from build123d import *

# Parameters (mm, degrees)
F0_W      = 1200
F0_H      = 400
F1_DEPTH  = 12
F2_W      = 38
F2_H      = 38
F3_DEPTH  = 128
F5_DEPTH  = 12
F7_DEPTH  = 25
F9_W      = 38
F9_H      = 38
F10_DEPTH = 120
F11_R     = 4
F12_DEPTH = 25
F13_W     = 1124
F13_H     = 324
F14_DEPTH = 25
F15_W     = 38
F15_H     = 116
F16_DEPTH = 19
F17_W     = 38
F17_H     = 116
F18_DEPTH = 19


with BuildPart() as f1:
    # F0 (on Top) → F1 (new body)
    with BuildSketch(Plane.XY):
        Rectangle(F0_W, F0_H)
    extrude(amount=F1_DEPTH)

    # F2 (on face) → F3 (join)
    with BuildSketch(Plane.XY.offset(12)):
        with Locations((-581, 181)):
            Rectangle(F2_W, F2_H)
        with Locations((581, 181)):
            Rectangle(F2_W, F2_H)
        with Locations((581, -181)):
            Rectangle(F2_W, F2_H)
        with Locations((-581, -181)):
            Rectangle(F2_W, F2_H)
    extrude(amount=F3_DEPTH)

    # F4 (on face) → F5 (join)
    with BuildSketch(Plane.XY.offset(140)):
        Polygon((600, 200), (-562, 200), (-562, 162), (-600, 162), (-600, -200), (600, -200), align=None)
    extrude(amount=-F5_DEPTH)

    # F6 (on face) → F7 (join)
    with BuildSketch(Plane.XZ.offset(200)):
        Polygon((-562, 128), (-562, 78), (-512, 128), align=None)
        Polygon((-512, 12), (-562, 62), (-562, 12), align=None)
        Polygon((562, 62), (512, 12), (562, 12), align=None)
        Polygon((562, 128), (512, 128), (562, 78), align=None)
    extrude(amount=-F7_DEPTH)

    # F8: F1 across plane


with BuildPart() as f1_1:
    add(f1.part)
    add(f1.part.mirror(Plane.XZ))

    # F9 (on face) → F10 (join)
    with BuildSketch(Plane.XY.offset(12)):
        with Locations((0, -181)):
            Rectangle(F9_W, F9_H)
        with Locations((0, 181)):
            Rectangle(F9_W, F9_H)
    extrude(amount=F10_DEPTH)

    # F11 (on face) → F12 (cut)
    with BuildSketch(Plane.XY.offset(12)):
        with Locations((-265.5, -181)):
            Circle(F11_R)
        with Locations((-581, 0)):
            Circle(F11_R)
        with Locations((-265.5, 185)):
            Circle(F11_R)
        with Locations((265.5, 181)):
            Circle(F11_R)
        with Locations((265.5, -181)):
            Circle(F11_R)
        with Locations((581, 0)):
            Circle(F11_R)
    extrude(amount=-F12_DEPTH, mode=Mode.SUBTRACT)

    # F13 (on face) → F14 (cut)
    with BuildSketch(Plane.XY.offset(140)):
        Rectangle(F13_W, F13_H)
    extrude(amount=-F14_DEPTH, mode=Mode.SUBTRACT)

    # F15 (on face) → F16 (cut)
    with BuildSketch(Plane.XZ.offset(200)):
        with Locations((0, 70)):
            Rectangle(F15_W, F15_H)
    extrude(amount=-F16_DEPTH, mode=Mode.SUBTRACT)

    # F17 (on face) → F18 (cut)
    with BuildSketch(Plane(origin=(0, 200, 0), x_dir=(-1, 0, 0), z_dir=(0, 1, 0))):
        with Locations((0, 70)):
            Rectangle(F17_W, F17_H)
    extrude(amount=-F18_DEPTH, mode=Mode.SUBTRACT)


solid = f1_1.part
Could you check a few things on this model? Use its own coordinates, in mm. A direction names the side the tool comes from. Give positions to 0.01 mm unless a question says otherwise; leave off trailing zeros. Order: outer loops, then holes, each group sorted by start corner. A loop starts at its lowest first (then second) coordinate and runs counter-clockwise, first axis right, second up. Notation, with made-up numbers: (36.25, 22.5) - (58.25, 22.5) arc R31 cw to (58.25, 47.5) - close; hole circle Ø2 at (-6.75, -5.5). An arc over 180 degrees is marked (long way). Return JSON: item names as keys, results as strings. Group by question number.
Q1. Which directions (+Z, -Z, +X, -X, +Y, -Y) give clear straight access to the entire face, cutting with the end or side of a thin tool? Please do faces 4 (the face through (-600, -3, 131)), 5 (the face through (-548, 175, 26)), 6 (the face through (581, 2, 128)), 7 (the face through (-537, 188, 103)).
Q2. Suppose I cut it at C-C, the plane x = -88. Please give me the cut outline in (y, z).
Q3. Suppose I cut it at B-B, the plane z = 44.5. State how many separate pieces and enclosed holes the cut face has, and give its area (3 significant figures).
Q4. Please list where these lines run through material, in increasing order: line 1 along Y through (x, z) = (-265.5, 5); line 2 along X through (y, z) = (177, 65.5); line 3 along Z through (x, y) = (107, -169). Write a range as [from, to].
Q5. Thinking about a two-plate mould opening in Y: for faces 1 (the face through (-537, 188, 37)), 2 (the face through (-8, 3, 12)), 3 (the face through (-3, -200, 132)), which applies, pulls with the +Y half, pulls with the -Y half, needs draft (parallel to the pull), parting line crosses it, or undercut?
Q6. Suppose I cut it at A-A, the plane y = -23.5. Please give me the cut outline in (x, z).
Q7. Will these pins go through, and if not, where does the flat tip stop? pin 1 Ø2 at (x, y) = (381.5, -106.5) entering from +Z; pin 2 Ø11.5 at (x, z) = (-7.5, 60) entering from +Y; pin 3 Ø1 at (x, y) = (-391, -150.5) entering from -Z.
Resolved:
{
 "1": {"face 4": "+Z, -Z, -X, +Y, -Y", "face 5": "none", "face 6": "+X, -X", "face 7": "+Y, -Y"},
 "2": {"outline": "(-200, 0) - (200, 0) - (200, 12) - (-200, 12) - close; (-200, 128) - (-162, 128) - (-162, 140) - (-200, 140) - close; (162, 128) - (200, 128) - (200, 140) - (162, 140) - close"},
 "3": {"separate pieces": "6", "enclosed holes": "0", "area": "8,970 mm2"},
 "4": {"line 1": "y = [-200, -185], [-177, 181], [189, 200]", "line 2": "x = [-600, -562], [-19, 19], [562, 600]", "line 3": "z = [0, 12], [128, 140]"},
 "5": {"face 1": "needs draft", "face 2": "undercut", "face 3": "pulls with the -Y half"},
 "6": {"outline": "(-600, 0) - (600, 0) - (600, 12) - (-600, 12) - close; (-600, 128) - (-562, 128) - (-562, 140) - (-600, 140) - close; (562, 128) - (600, 128) - (600, 140) - (562, 140) - close"},
 "7": {"pin 1": "stops at z = 12", "pin 2": "stops at y = 181", "pin 3": "stops at z = 0"}
}
